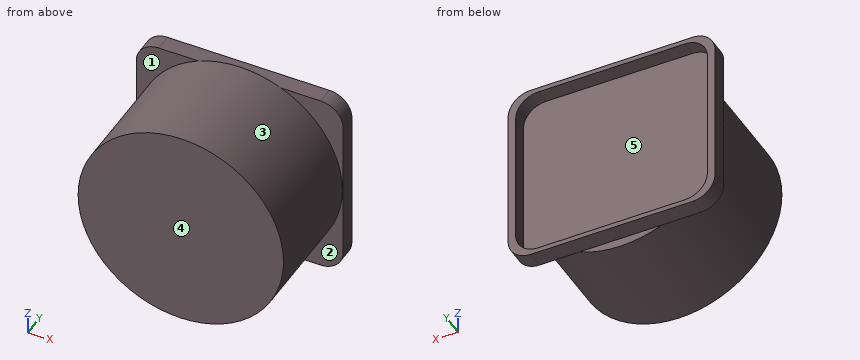
from build123d import *

# Parameters (mm, degrees)
BOSS_EXTRUDE1_DEPTH = 2.032
BOSS_EXTRUDE2_DEPTH = 0.254
SKETCH3_R           = 13.87475
BOSS_EXTRUDE3_DEPTH = 15.35


with BuildPart() as part:
    # Sketch1 → Boss-Extrude1 (new body)
    with BuildSketch(Plane(origin=(0, 0, 0), x_dir=(1, 0, 0), z_dir=(0, 1, 0))):
        with BuildLine():
            Line((-10.922, -12.7), (10.922, -12.7))
            ThreePointArc((10.922, -12.7), (13.077261469, -11.807261469), (13.97, -9.652))
            Line((13.97, -9.652), (13.97, 9.652))
            ThreePointArc((13.97, 9.652), (13.077261469, 11.807261469), (10.922, 12.7))
            Line((10.922, 12.7), (-10.922, 12.7))
            ThreePointArc((-10.922, 12.7), (-13.077261469, 11.807261469), (-13.97, 9.652))
            Line((-13.97, 9.652), (-13.97, -9.652))
            ThreePointArc((-13.97, -9.652), (-13.077261469, -11.807261469), (-10.922, -12.7))
        make_face()
        with BuildLine():
            Line((-9.906, -12.065), (9.906, -12.065))
            ThreePointArc((9.906, -12.065), (12.061261469, -11.172261469), (12.954, -9.017))
            Line((12.954, -9.017), (12.954, 9.017))
            ThreePointArc((12.954, 9.017), (12.061261469, 11.172261469), (9.906, 12.065))
            Line((9.906, 12.065), (-9.906, 12.065))
            ThreePointArc((-9.906, 12.065), (-12.061261469, 11.172261469), (-12.954, 9.017))
            Line((-12.954, 9.017), (-12.954, -9.017))
            ThreePointArc((-12.954, -9.017), (-12.061261469, -11.172261469), (-9.906, -12.065))
        make_face(mode=Mode.SUBTRACT)
    extrude(amount=BOSS_EXTRUDE1_DEPTH)

    # Sketch2 → Boss-Extrude2 (add)
    with BuildSketch(Plane.XZ):
        with BuildLine():
            Line((-10.922, -12.7), (10.922, -12.7))
            ThreePointArc((10.922, -12.7), (13.077261469, -11.807261469), (13.97, -9.652))
            Line((13.97, -9.652), (13.97, 9.652))
            ThreePointArc((13.97, 9.652), (13.077261469, 11.807261469), (10.922, 12.7))
            Line((10.922, 12.7), (-10.922, 12.7))
            ThreePointArc((-10.922, 12.7), (-13.077261469, 11.807261469), (-13.97, 9.652))
            Line((-13.97, 9.652), (-13.97, -9.652))
            ThreePointArc((-13.97, -9.652), (-13.077261469, -11.807261469), (-10.922, -12.7))
        make_face()
    extrude(amount=BOSS_EXTRUDE2_DEPTH)

    # Sketch3 → Boss-Extrude3 (add)
    with BuildSketch(Plane.XZ.offset(0.254)):
        Circle(SKETCH3_R)
    extrude(amount=BOSS_EXTRUDE3_DEPTH)


solid = part.part
Design review of the part built by this model. Coordinates are the model's own, in mm. Face numbers are marked on the shaded views. A direction names the side the tool comes from. Coordinates: 2 decimals unless noted, no trailing zeros. Order: outer loops, then holes, each group sorted by start corner. A loop starts at its lowest first (then second) coordinate and runs counter-clockwise, first axis right, second up. Notation, with made-up numbers: (-18.5, -5) -> (28.5, -5) arc R24 cw to (28.5, 26) -> close; hole circle Ø6 at (21.5, 40). An arc over 180 degrees is marked (long way). Use one line per item in the form item = value. Start each with the question number.
(1) Add section C-C on y = -8.5. State the section outline as (x, z) points.
(2) For probe 1 along Z at (x, y) = (-8.25, 0.5) (3 decimals); probe 2 along X at (y, z) = (0.5, -7); probe 3 along Y at (x, z) = (-7.25, -10.5), list the stretches that pass through material, from the lowest coordinate up.
(3) The part is to be moulded in two halves that separate along X. For the marked faces 3, 4 and 5, say which applies: +X half, -X half, draft (parallel to the pull), parting line (faces both ways), or undercut.
(4) Insertion check: pin 1 (1.8 mm diameter, centred on x = -4, y = 1.5, fed in from -Z); pin 2 (10 mm diameter, centred on y = -12, z = -5, fed in from -X); pin 3 (1.3 mm diameter, centred on x = -2.5, z = -13.5, fed in from +Y). Each pin has a flat end and moves straight along its axis. Give the tip position at first contact, or say it passes through.
(5) For the marked faces 1 and 2, list the 3-axis set-ups (+Z, -Z, +X, -X, +Y, -Y) from which the entire face can be reached by the end or side of a thin tool; tool diameter is ignored.
(6) Add section A-A on z = 0. State the section outline as (x, y) points.
(7) Add section B-B on x = 0. State the section outline as (y, z) points (3 decimals), plus the area to 3 significant figures.
Answer block:
q1.outline = circle Ø27.75 at (0, 0)
q2.probe_1 = -12.7 to -12.065, 12.065 to 12.7
q2.probe_2 = -13.97 to -12.95, 12.95 to 13.97
q2.probe_3 = -15.6 to 0
q3.face_3 = parting line
q3.face_4 = draft
q3.face_5 = undercut
q4.pin_1 = -12.7
q4.pin_2 = -13.87
q4.pin_3 = -0.25
q5.face_1 = -X, -Y
q5.face_2 = +X, -Y
q6.outline = (-13.97, -0.25) -> (-13.87, -0.25) -> (-13.87, -15.6) -> (13.87, -15.6) -> (13.87, -0.25) -> (13.97, -0.25) -> (13.97, 2.03) -> (12.95, 2.03) -> (12.95, 0) -> (-12.95, 0) -> (-12.95, 2.03) -> (-13.97, 2.03) -> close
q7.outline = (-15.604, -13.875) -> (-0.254, -13.875) -> (-0.254, -12.7) -> (2.032, -12.7) -> (2.032, -12.065) -> (0, -12.065) -> (0, 12.065) -> (2.032, 12.065) -> (2.032, 12.7) -> (-0.254, 12.7) -> (-0.254, 13.875) -> (-15.604, 13.875) -> close
q7.area = 435 mm²
